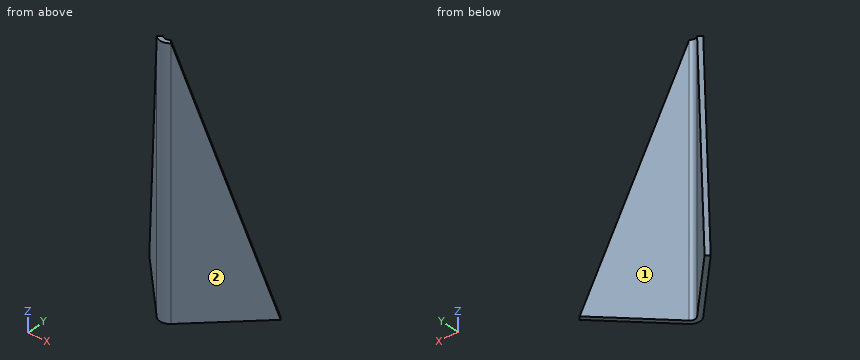
from build123d import *

# Parameters (mm, degrees)
BASE_FLANGE1_DEPTH = 55
CUT_EXTRUDE1_DEPTH = 10
CUT_EXTRUDE2_DEPTH = 10


# Read off the part's stored shape, not the designer's step: Base-Flange1
with BuildPart() as part:
    # Base-Flange1 outline → Base-Flange1 (new body)
    with BuildSketch(Plane.XY):
        with BuildLine():
            Line((-0.848528137, 2.2627417), (-13.435028843, 14.849242405))
            Line((-13.435028843, 14.849242405), (-14.142135624, 14.142135624))
            Line((-14.142135624, 14.142135624), (-1.555634919, 1.555634919))
            ThreePointArc((-1.555634919, 1.555634919), (0, 0.911269837), (1.555634919, 1.555634919))
            Line((1.555634919, 1.555634919), (14.142135624, 14.142135624))
            Line((14.142135624, 14.142135624), (13.435028843, 14.849242405))
            Line((13.435028843, 14.849242405), (0.848528137, 2.2627417))
            ThreePointArc((0.848528137, 2.2627417), (0, 1.911269837), (-0.848528137, 2.2627417))
        make_face()
    extrude(amount=BASE_FLANGE1_DEPTH)

    # Sketch6 → Cut-Extrude1 (cut)
    with BuildSketch(Plane(origin=(0, 0, 0), x_dir=(0, 0, 1), z_dir=(-0.7071067811865477, -0.7071067811865475, 0))):
        Polygon((0, 20), (55, 2.2), (55, 20), align=None)
    extrude(amount=-CUT_EXTRUDE1_DEPTH, mode=Mode.SUBTRACT)

    # Sketch7 → Cut-Extrude2 (cut)
    with BuildSketch(Plane(origin=(0, 0, 0), x_dir=(0, 0, -1), z_dir=(0.7071067811865488, -0.7071067811865462, 0))):
        Polygon((-55, 2.2), (0, 20), (-55, 20), align=None)
    extrude(amount=-CUT_EXTRUDE2_DEPTH, mode=Mode.SUBTRACT)


solid = part.part
Could you check a few things on this model? Use its own coordinates, in mm. Face numbers are marked on the shaded views. Round coordinates to 2 decimals unless told otherwise and drop trailing zeros. Loops run counter-clockwise (first coordinate to the right, second up) from the corner with the lowest first, then second, coordinate; pieces in that order, holes last. Notation, with made-up numbers: (50.25, 87.5) - (68.25, 87.5) arc R8 ccw to (68.25, 91.5) - close; hole circle Ø11 at (75, 40.5). An arc over 180 degrees is marked (long way). Write item = value, one per line.
1) Imagine slicing it at C-C (y = 12.75). Please give me the cut outline in (x, z).
Computed:
outline = (-12.75, 0) - (-11.34, 0) - (-11.34, 9.17) - (-12.75, 6.08) - close; (11.34, 0) - (12.75, 0) - (12.75, 6.08) - (11.34, 9.17) - close
2) Imagine slicing it at D-D (z = 37). Please give me the cut outline in (x, y), and give its area (3 significant figures).
Computed:
outline = (-5.67, 5.67) - (-1.56, 1.56) arc R2.2 ccw to (1.56, 1.56) - (5.67, 5.67) - (4.97, 6.38) - (0.85, 2.26) arc R1.2 cw to (-0.85, 2.26) - (-4.97, 6.38) - close
area = 14.3 mm2
3) Imagine slicing it at B-B (z = 26). Please give me the cut outline in (x, y).
Computed:
outline = (-8.19, 8.19) - (-1.56, 1.56) arc R2.2 ccw to (1.56, 1.56) - (8.19, 8.19) - (7.49, 8.9) - (0.85, 2.26) arc R1.2 cw to (-0.85, 2.26) - (-7.49, 8.9) - close
4) If we mould it in two halves opening along X, with no side actions, what happens to the marked faces 1 and 2? For each: pulls with the +X half, pulls with the -X half, needs draft (parallel to the pull), parting line crosses it, or undercut.
Computed:
face_1 = undercut
face_2 = pulls with the +X half
5) I need wall thicknesses on line 1 along Y through (x, z) = (8, 7.5); line 2 along Y through (x, z) = (-2.5, 43); line 3 along X through (y, z) = (7, 19). Which ranges of each line are inside material? Lowest first, please. Write a range as from..to.
Computed:
line_1 = 8..9.41
line_2 = 2.5..3.91
line_3 = -7..-5.59, 5.59..7
6) Imagine slicing it at A-A (y = 9). Please give me the cut outline in (x, z), and give its area (3 significant figures).
Computed:
outline = (-9, 0) - (-7.59, 0) - (-7.59, 25.56) - (-9, 22.47) - close; (7.59, 0) - (9, 0) - (9, 22.47) - (7.59, 25.56) - close
area = 67.9 mm2
7) I'm going to push flat-ended pins straight in: P1, Ø1.5, axis at x = 7, z = 25, coming from the -Y side; P2, Ø1.5, axis at y = 8, z = 8.5, coming from the +X side; P3, Ø2, axis at x = -5, z = 27, coming from the +Y side; P4, Ø1.5, axis at x = -7.5, y = 4.5, coming from the +Z side. Where does each tip first touch, or does it pass through?
Computed:
P1 = 6.25
P2 = 8.75
P3 = 7.41
P4 = through
